The listing builds one solid part. Answer for the finished solid, in the listing's coordinates (mm). Face numbers are marked on the shaded views. A direction names the side the tool comes from. Round coordinates to 2 decimals unless told otherwise and drop trailing zeros. Order: outer loops, then holes, each group sorted by start corner. A loop starts at its lowest first (then second) coordinate and runs counter-clockwise, first axis right, second up. Notation, with made-up numbers: (22, 32) - (51, 32) arc R30 ccw to (51, 70) - close; hole circle Ø3 at (31.5, -8). An arc over 180 degrees is marked (long way). Use CSV: the item, a comma, the result in double quotes. Start each with the question number.
Item 1: Find section C-C, the plane x = 18. Give the vertices of the cut face in (y, z), plus the area to 3 significant figures.
Item 2: For the marked faces 1 and 2, determine the directions among +Z, -Z, +X, -X, +Y, -Y from which every point of the face is accessible in a straight line to the end or side of a thin tool.
Item 3: Straight lines are drawn through the part: line 1 along Z through (x, y) = (8.75, -3.25); line 2 along X through (y, z) = (-2.25, -22); line 3 along Z through (x, y) = (5.25, -11). For each, find the intervals that lie inside material, in ascending order. Write a range as [from, to].
Item 4: Find section B-B, the plane z = -22. Give the vertices of the cut face in (x, y).
Item 5: Find section A-A, the plane y = 12.5. Give the vertices of the cut face in (x, z), plus the area to 3 significant figures.
Item 6: A flat-ended cylindrical pin translates along its axis: P1, Ø7, axis at x = 16, y = 5.5, coming from the +Z side. Find the tip coordinate at first contact, or state that the pin passes through.
```python
from build123d import *

# Parameters (mm, degrees)
SKETCH3_W = 3
SKETCH3_H = 30
FILLET1_R = 3.2
FILLET2_R = 6.4


with BuildPart() as part:
    # Sweep1: sweep along a path in Sketch4
    with BuildLine(Plane(origin=(0, 0, 0), x_dir=(1, 0, 0), z_dir=(0, 1, 0))) as sweep1_path:
        Line((0, 0), (0, 35))
        Line((0, 35), (30, 35))
    # Sketch3 → Sweep1 (sweep)
    with BuildSketch(Plane.XY):
        with Locations((1.5, 0)):
            Rectangle(SKETCH3_W, SKETCH3_H)
    sweep(path=sweep1_path.line, transition=Transition.RIGHT)

    # Fillet1
    fillet1_edges = [part.edges().sort_by_distance(p)[0] for p in [
        (3, 0, -32),
    ]]
    fillet(fillet1_edges, radius=FILLET1_R)

    # Fillet2
    fillet2_edges = [part.edges().sort_by_distance(p)[0] for p in [
        (0, 0, -35),
    ]]
    fillet(fillet2_edges, radius=FILLET2_R)


solid = part.part
```
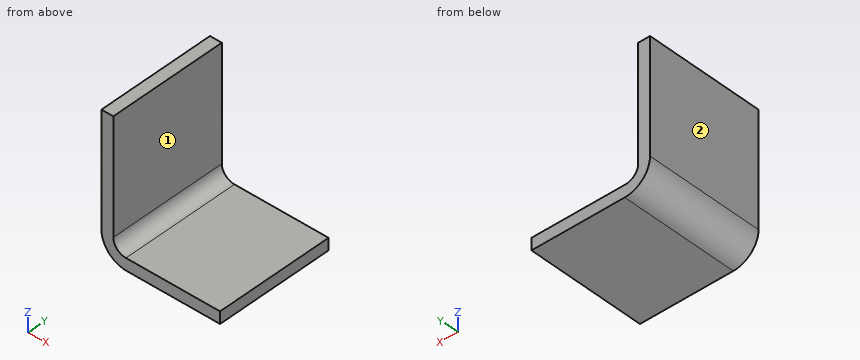
Worked out:
1,outline,"(-15, -35) - (15, -35) - (15, -32) - (-15, -32) - close"
1,area,"90.0 mm²"
2,face 1,"+Z, +X, +Y, -Y"
2,face 2,"+Z, -Z, -X, +Y, -Y"
3,line 1,"z = [-35, -32]"
3,line 2,"x = [0, 3]"
3,line 3,"z = [-34.9, -31.86]"
4,outline,"(0, -15) - (3, -15) - (3, 15) - (0, 15) - close"
5,outline,"(0, -28.6) arc R6.4 ccw to (6.4, -35) - (30, -35) - (30, -32) - (6.2, -32) arc R3.2 cw to (3, -28.8) - (3, 0) - (0, 0) - close"
5,area,"179 mm²"
6,P1,"stops at z = -32"
